Read the model definition and answer for the solid it produces. Units are mm, in the model's axes. Give positions to 0.01 mm unless a question says otherwise; leave off trailing zeros. Order: outer loops, then holes, each group sorted by start corner. A loop starts at its lowest first (then second) coordinate and runs counter-clockwise, first axis right, second up. Notation, with made-up numbers: (33, 75.5) -> (41, 75.5) arc R19 ccw to (41, 111.5) -> close; hole circle Ø2 at (-1.75, 12.5). An arc over 180 degrees is marked (long way). Use one line per item in the form item = value.
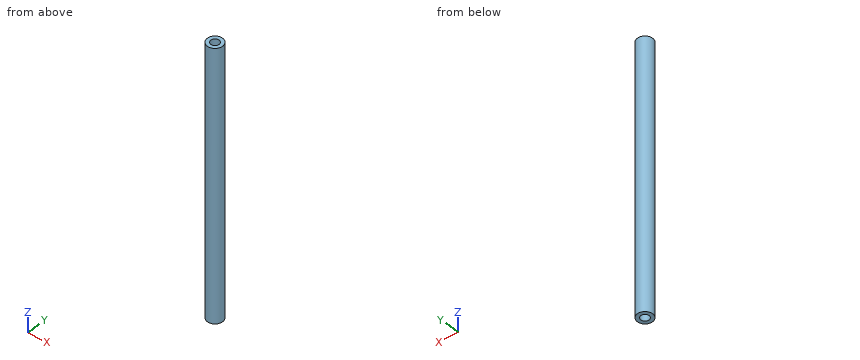
```python
from build123d import *

# Parameters (mm, degrees)
SKETCH1_R                              = 6.35
BOSS_EXTRUDESHAFT_DEPTH                = 111
BOSS_EXTRUDESHAFT_DEPTH_BACK           = 111
F_5_16_24_TAPPED_HOLE2_D               = 6.9088
F_5_16_24_TAPPED_HOLE2_DEPTH           = 40
F_5_16_24_TAPPED_HOLE2_TIP             = 2.075612922
F_5_16_24_TAPPED_HOLE2_ON_FACE_2_D     = 6.9088
F_5_16_24_TAPPED_HOLE2_ON_FACE_2_DEPTH = 40
F_5_16_24_TAPPED_HOLE2_ON_FACE_2_TIP   = 2.075612922


with BuildPart() as part:
    # Sketch1 → Boss-ExtrudeShaft (new body, two sides)
    with BuildSketch(Plane.XY) as boss_extrudeshaft_sk:
        Circle(SKETCH1_R)
    extrude(amount=BOSS_EXTRUDESHAFT_DEPTH)
    extrude(boss_extrudeshaft_sk.sketch, amount=-BOSS_EXTRUDESHAFT_DEPTH_BACK)

    # 5_16-24 Tapped Hole2
    with Locations(Plane(origin=(0, 0, -111), x_dir=(-1, 0, 0), z_dir=(0, 0, -1))):
        with Locations((0, 0)):
            Hole(F_5_16_24_TAPPED_HOLE2_D / 2, depth=F_5_16_24_TAPPED_HOLE2_DEPTH)
            with Locations((0, 0, -(F_5_16_24_TAPPED_HOLE2_DEPTH + F_5_16_24_TAPPED_HOLE2_TIP / 2))):  # 118° drill point
                Cone(0, F_5_16_24_TAPPED_HOLE2_D / 2, F_5_16_24_TAPPED_HOLE2_TIP, mode=Mode.SUBTRACT)

    # 5_16-24 Tapped Hole2 on face 2
    with Locations(Plane.XY.offset(111)):
        with Locations((0, 0)):
            Hole(F_5_16_24_TAPPED_HOLE2_ON_FACE_2_D / 2, depth=F_5_16_24_TAPPED_HOLE2_ON_FACE_2_DEPTH)
            with Locations((0, 0, -(F_5_16_24_TAPPED_HOLE2_ON_FACE_2_DEPTH + F_5_16_24_TAPPED_HOLE2_ON_FACE_2_TIP / 2))):  # 118° drill point
                Cone(0, F_5_16_24_TAPPED_HOLE2_ON_FACE_2_D / 2, F_5_16_24_TAPPED_HOLE2_ON_FACE_2_TIP, mode=Mode.SUBTRACT)


solid = part.part
```
Item 1: The part is cut by section B-B on z = 22.5. Give the vertices of the cut face in (x, y), and give its area (3 significant figures).
Checks:
outline = circle Ø12.7 at (0, 0)
area = 127 mm²
Item 2: The part is cut by section A-A on z = -74. Give the vertices of the cut face in (x, y).
Checks:
outline = circle Ø12.7 at (0, 0); hole circle Ø6.91 at (0, 0)
Item 3: Given pin 1 Ø5 at (y, z) = (-4.5, -8) entering from -X; pin 2 Ø5 at (x, z) = (-3, -43) entering from -Y; pin 3 Ø6 at (x, y) = (0, 0) entering from +Z, each flat-ended and moving along its own axis, determine where each tip first touches the part or whether it passes through.
Checks:
pin_1 = -6.03
pin_2 = -6.33
pin_3 = 70.73
Item 4: Straight lines are drawn through the part: L1, parallel to Y at x = 0, z = 88.5; L2, parallel to Y at x = 2.5, z = 99.5; L3, parallel to X at y = 5, z = 54. For each, find the intervals that lie inside material, in ascending order. Write a range as from..to.
Checks:
L1 = -6.35..-3.45, 3.45..6.35
L2 = -5.84..-2.38, 2.38..5.84
L3 = -3.91..3.91
